Autodesk Inventor part; units mm, degrees
ref_plane "Work Plane1" through (-8.8582, 0, 0) normal (0, -0.866, -0.5) x (1, 0, 0)
ref_plane "YZ Plane" through (0, 0, 0) normal (1, 0, 0) x (0, 1, 0)
ref_plane "XZ Plane" through (0, 0, 0) normal (0, 1, 0) x (-1, 0, 0)
sketch "Sketch1" plane through (0, 0, 0) normal (1, 0, 0) x (0, 1, 0)
  line L0 (-4.6188, 0) -> (-2.3094, 4)
  line L1 (-2.3094, 4) -> (2.3094, 4)
  line L2 (2.3094, 4) -> (4.6188, 0)
  line L3 (4.6188, 0) -> (2.3094, -4)
  line L4 (2.3094, -4) -> (-2.3094, -4)
  line L5 (-2.3094, -4) -> (-4.6188, 0)
  point P0 (0, 0)
  point P1 (0, 0)
  dimension "d0" = 9.2376
extrude "Body" add sketch "Sketch1" along normal blind 4
sketch "Sketch2" plane through (0, 0, 0) normal (0, 0, 1) x (1, 0, 0)
  line L0 (0, 2.3094) -> (0, 4.6188)
  line L1 (0, 4.6188) -> (4, 4.6188)
  line L2 (4, 2.3094) -> (4, 4.6188)
  line L3 (-0.8, 0) -> (4.8, 0)
  line L4 (0.3573, 4.6188) -> (0, 4)
  line L5 (3.6427, 4.6188) -> (4, 4)
  dimension "d3" = 30
  dimension "d4" = 30
  dimension "d5" = 8
  dimension "d6" = 8
revolve "Chamfer1" cut sketch "Sketch2" angle 360 about axis through (-10, 0, 0) along (1, 0, 0)
sketch "Sketch3" plane through (4, 0, 0) normal (1, 0, 0) x (0, 0, -1)
  arc A0 (-2, -3.4641) -> (2, -3.4641) centre (0, 0) ccw
hole "Thread" at (4, 0, 0) direction (-1, 0, 0) diameter 4.134 end through all
chamfer "Chamfer2" distance 0.433 angle 30 1 edges at (4, 0, 2.067) measured on face at (4, 3.336, -0.083)
chamfer "Chamfer3" distance 0.433 angle 30 1 edges at (0, 0, 2.067) measured on face at (0, 3.336, -0.083)
ref_plane "Work Plane1" through (-8.8582, 0, 0) normal (0, -0.866, -0.5) x (1, 0, 0)
equation "\"d0\" = 1.1547 * SW"
equation "\"d1\" = KOH"
equation "\"d3\" = ANG1"
equation "\"d4\" = ANG2"
equation "\"d5\" = SW0"
equation "\"d6\" = SW01"
equation "\"d8\" = -0.5 * GD1 + 0.5 * NND"
equation "\"d40\" = -0.5 * GD1 + 0.5 * NND"
equation "\"d10\" = -0.5 * GD1 + 0.5 * NND"
equation "\"d41\" = -0.5 * GD1 + 0.5 * NND"
equation "\"ANG1\" = 30deg"
equation "\"ANG2\" = 30deg"
equation "\"NND\" = 5"
equation "\"KOH\" = 4"
equation "\"SW\" = 8"
equation "\"SW0\" = SW"
equation "\"SW01\" = SW"
equation "\"GUL\" = 0.541266 * PTC"
equation "\"THREADDIA\" = 5"
equation "\"TOA\" = 30deg"
equation "\"PTC\" = 0.8"
equation "\"E0\" = 1.155 * SW"
equation "\"GAL\" = 0.541266 * PTC"
properties part number "JIS B 1181 - HN - Class 2 Finished M5" material "Steel, Mild"
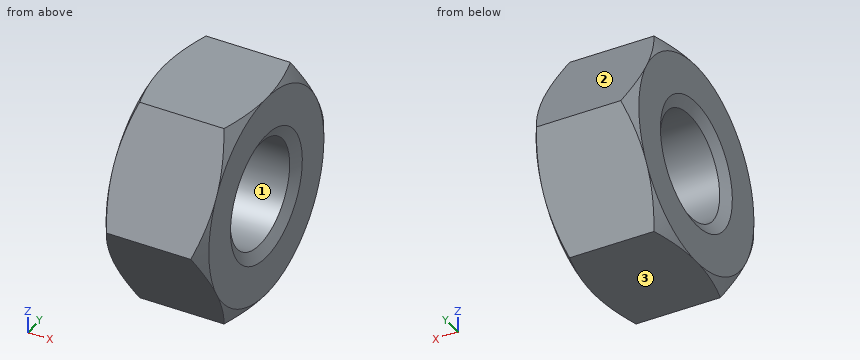
The listing builds one solid part. Answer for the finished solid, in the listing's coordinates (mm). Face numbers are marked on the shaded views. Coordinates: 2 decimals unless noted, no trailing zeros. Loops run counter-clockwise (first coordinate to the right, second up) from the corner with the lowest first, then second, coordinate; pieces in that order, holes last. Notation, with made-up numbers: M 14,10.5 L 61,10.5 A30 ccw 61,42.5 Z; hole C 63,-18 d11. An arc over 180 degrees is marked long. Answer in a Markdown table with one row per item.
1) Find the intervals of material crossed by probe 1 along Z at (x, y) = (1.65, 0); probe 2 along Z at (x, y) = (3.5, 0.5); probe 3 along Y at (x, z) = (2.3, 1.25), in increasing order.
Answers below:
| item | result |
|---|---|
| probe 1 | -4 to -2.07, 2.07 to 4 |
| probe 2 | -4 to -2.01, 2.01 to 4 |
| probe 3 | -3.9 to -1.65, 1.65 to 3.9 |
2) Determine the mould class of the marked faces 1, 2 and 3 for opening direction Z: released by +Z, released by -Z, zero draft, split by the parting line, or undercut.
Answers below:
| item | result |
|---|---|
| face 1 | undercut |
| face 2 | released by +Z |
| face 3 | released by -Z |
3) Find section A-A (x = 3.25). Determine the outline of the cut face in (y, z).
Answers below:
| item | result |
|---|---|
| outline | M -4.62,0 L -2.31,-4 L 2.31,-4 L 4.62,0 L 2.31,4 L -2.31,4 Z; hole C 0,0 d4.13 |
4) Given pin 1 (2 mm diameter, centred on x = 2.5, y = -3.5, fed in from -Z); pin 2 (3.5 mm diameter, centred on y = 0, z = 0, fed in from +X), each flat-ended and moving along its own axis, determine where each tip first touches the part or whether it passes through.
Answers below:
| item | result |
|---|---|
| pin 1 | z = -3.67 |
| pin 2 | through |
